The listing builds one solid part. Answer for the finished solid, in the listing's coordinates (mm). A direction names the side the tool comes from. Give positions to 0.01 mm unless a question says otherwise; leave off trailing zeros. Write each loop counter-clockwise with the first axis right and the second up, starting at its lowest first coordinate (ties: lowest second). Pieces come first, ordered by that corner, then holes. Notation, with made-up numbers: (-12, -29) -> (45, -29) arc R7 ccw to (45, -16) -> close; hole circle Ø11 at (15.25, -37.75). An arc over 180 degrees is marked (long way). Put each result on its own line as item: value. Start each with the question number.
1) A cutting plane is placed at C-C (z = -9.75). Write down the section's boundary in (x, y), then the cut area to 3 significant figures.
2) For a pull along Z with two mould halves and no side action, classify faces 5 (the cylindrical face through (-8.9, 2.5, 0.1)), 6 (the flat face through (3, 5, -2)), 7 (the cylindrical face through (-7.286, 2.465, 0.575)), 8 (the flat face through (0, 2, -12)) as released by +Z, released by -Z, zero draft, split by the parting line, or undercut.
3) For faces 1 (the flat face through (-4.25, 2, -9)), 2 (the flat face through (-4.25, 2, 7)), 3 (the flat face through (4.25, 2, 8)), 4 (the flat face through (4.25, 2, -8)), determine the directions among +Z, -Z, +X, -X, +Y, -Y from which every point of the face is accessible in a straight line to the end or side of a thin tool.
4) A cutting plane is placed at A-A (y = 2.75). Write down the section's boundary in (x, z), then the cut area to 3 significant figures.
5) Flat-ended cylindrical pins translate along their axes: pin 1 Ø2.5 at (y, z) = (3.5, -9.5) entering from -X; pin 2 Ø1.3 at (x, y) = (0.5, 2) entering from +Z; pin 3 Ø1 at (y, z) = (2, -1) entering from -X; pin 4 Ø2.5 at (x, z) = (5.9, 0) entering from +Y. Find the tip coordinate at first contact, or state that the pin passes through.
6) A cutting plane is placed at B-B (z = 0). Write down the section's boundary in (x, y).
7) Find the intervals of material crossed by line 1 along X through (y, z) = (3.2, -9.5); line 2 along X through (y, z) = (1.9, -0.75); line 3 along Z through (x, y) = (-1.75, 4.25), in increasing order. Write a range as from..to.
8) A cutting plane is placed at D-D (z = 4.75). Write down the section's boundary in (x, y).
Autodesk Inventor part; units mm, degrees
ref_plane "YZ Plane" through (0, 0, 0) normal (1, 0, 0) x (0, 1, 0)
ref_plane "XZ Plane" through (0, 0, 0) normal (0, 1, 0) x (-1, 0, 0)
ref_plane "XY Plane" through (0, 0, 0) normal (0, 0, 1) x (1, 0, 0)
sketch "Sketch1" plane through (0, 0, 0) normal (0, 1, 0) x (-1, 0, 0)
  line L0 (2.25, 10) -> (-2.25, 10)
  line L1 (-2.25, 10) -> (-2.25, -10)
  line L2 (-2.25, -10) -> (2.25, -10)
  line L3 (2.25, -10) -> (2.25, 10)
  line L4 (4.25, 10) -> (-4.25, 10)
  line L5 (-4.25, -12) -> (4.25, -12)
  circle A0 centre (5.9, 0) radius 1.5
  circle A1 centre (-5.9, 0) radius 1.5
  arc A2 (-4.25, 2.5055) -> (-4.25, -2.5055) centre (-5.9, 0) ccw
  arc A3 (4.25, -2.5055) -> (4.25, 2.5055) centre (5.9, 0) ccw
  line L6 (4.25, -12) -> (4.25, -2.5055)
  line L7 (4.25, 2.5055) -> (4.25, 10)
  line L8 (-4.25, 10) -> (-4.25, 2.5055)
  line L9 (-4.25, -2.5055) -> (-4.25, -12)
  point P0 (0, 0)
  point P1 (0, -12)
  point P2 (0, -10)
  point P3 (2.25, 0)
  dimension "d0" = 4.5
  dimension "d1" = 20
  dimension "d2" = 5.9
  dimension "d3" = 11.8
  dimension "d4" = 3
  dimension "d5" = 3
  dimension "d6" = 6
  dimension "d7" = 6
  dimension "d8" = 2
  dimension "d9" = 2
  dimension "d10" = 2
  dimension "d11" = 2
extrude "Extrusion1" add sketch "Sketch1" along normal blind 5 contours L4 L7 A3 L6 L5 L9 A2 L8 L1 L2 L3
fillet "Fillet1" radius 2 4 edges at (4.25, 2.5, 2.5055) (-4.25, 2.5, 2.5055) (-4.25, 2.5, -2.5055) (4.25, 2.5, -2.5055)
properties part number "Stand Clamp"
Reply:
1. outline: (-4.25, 0) -> (-2.25, 0) -> (-2.25, 5) -> (-4.25, 5) -> close; (2.25, 0) -> (4.25, 0) -> (4.25, 5) -> (2.25, 5) -> close
1. area: 20.0 mm2
2. face 5: split by the parting line
2. face 6: zero draft
2. face 7: undercut
2. face 8: released by -Z
3. face 1: -Z, -X, +Y, -Y
3. face 2: +Z, -X, +Y, -Y
3. face 3: +Z, +X, +Y, -Y
3. face 4: -Z, +X, +Y, -Y
4. outline: (-6.11, -2.99) arc R2 cw to (-4.25, -4.99) -> (-4.25, -12) -> (4.25, -12) -> (4.25, -4.99) arc R2 cw to (6.11, -2.99) arc R3 ccw to (6.11, 2.99) arc R2 cw to (4.25, 4.99) -> (4.25, 10) -> (2.25, 10) -> (2.25, -10) -> (-2.25, -10) -> (-2.25, 10) -> (-4.25, 10) -> (-4.25, 4.99) arc R2 cw to (-6.11, 2.99) arc R3 ccw to start; hole circle Ø3 at (-5.9, 0); hole circle Ø3 at (5.9, 0)
4. area: 134 mm2
5. pin 1: stops at x = -4.25
5. pin 2: stops at z = -10
5. pin 3: stops at x = -8.86
5. pin 4: passes through
6. outline: (-8.9, 0) -> (-7.4, 0) -> (-7.4, 5) -> (-8.9, 5) -> close; (-4.4, 0) -> (-2.25, 0) -> (-2.25, 5) -> (-4.4, 5) -> close; (2.25, 0) -> (4.4, 0) -> (4.4, 5) -> (2.25, 5) -> close; (7.4, 0) -> (8.9, 0) -> (8.9, 5) -> (7.4, 5) -> close
7. line 1: x = -4.25..-2.25, 2.25..4.25
7. line 2: x = -8.8..-7.2, -4.6..-2.25, 2.25..4.6, 7.2..8.8
7. line 3: z = -12..-10
8. outline: (-4.26, 0) -> (-2.25, 0) -> (-2.25, 5) -> (-4.26, 5) -> close; (2.25, 0) -> (4.26, 0) -> (4.26, 5) -> (2.25, 5) -> close
